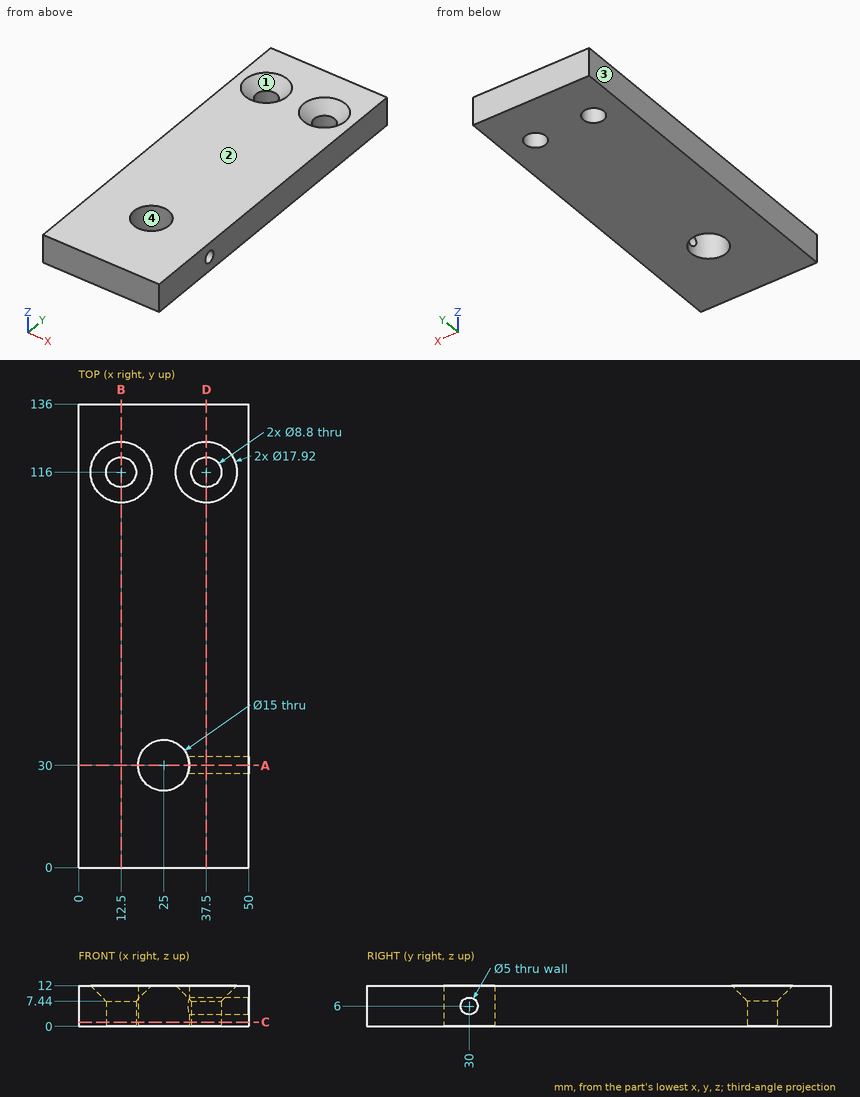
Here's the drawing with two shaded views (mm, measured from the low corner). I have some questions. Round coordinates to 2 decimals unless told otherwise and drop trailing zeros. Order: outer loops, then holes, each group sorted by start corner. A loop starts at its lowest first (then second) coordinate and runs counter-clockwise, first axis right, second up. Notation, with made-up numbers: (-32, 57.25) -> (14, 57.25) arc R25 cw to (14, 90.25) -> close; hole circle Ø1 at (-17, 27). An arc over 180 degrees is marked (long way). Return JSON: item names as keys, results as strings.
Q1. If we section it at A-A on y = 30: List the corners of the cut face in (x, z) for me.
Filled sheet:
{"outline": "(0, 0) -> (17.5, 0) -> (17.5, 12) -> (0, 12) -> close; (32.5, 0) -> (50, 0) -> (50, 3.5) -> (32.5, 3.5) -> close; (32.5, 8.5) -> (50, 8.5) -> (50, 12) -> (32.5, 12) -> close"}
Q2. If we mould it in two halves opening along X, with no side actions, what happens to the marked faces 1, 2, 3 and 4? For each: released by +X, released by -X, zero draft, split by the parting line, or undercut.
Filled sheet:
{"face 1": "undercut", "face 2": "zero draft", "face 3": "released by -X", "face 4": "undercut"}
Q3. If we section it at B-B on x = 12.5: List the corners of the cut face in (y, z) for me.
Filled sheet:
{"outline": "(0, 0) -> (111.6, 0) -> (111.6, 7.44) -> (107.04, 12) -> (0, 12) -> close; (120.4, 0) -> (136, 0) -> (136, 12) -> (124.96, 12) -> (120.4, 7.44) -> close"}
Q4. If we section it at D-D on x = 37.5: List the corners of the cut face in (y, z) for me, plus the area to 3 significant figures.
Filled sheet:
{"outline": "(0, 0) -> (111.6, 0) -> (111.6, 7.44) -> (107.04, 12) -> (0, 12) -> close; (120.4, 0) -> (136, 0) -> (136, 12) -> (124.96, 12) -> (120.4, 7.44) -> close; hole circle Ø5 at (30, 6)", "area": "1,490 mm^2"}
Q5. I need wall thicknesses on line 1 along X through (y, z) = (116, 4); line 2 along Z through (x, y) = (44.5, 30); line 3 along Y through (x, z) = (24.5, 1.75). Which ranges of each line are inside material? Lowest first, please. Write a range as from..to.
Filled sheet:
{"line 1": "x = 0..8.1, 16.9..33.1, 41.9..50", "line 2": "z = 0..3.5, 8.5..12", "line 3": "y = 0..22.52, 37.48..136"}
Q6. If we section it at C-C on z = 1.25: List the corners of the cut face in (x, y) for me.
Filled sheet:
{"outline": "(0, 0) -> (50, 0) -> (50, 136) -> (0, 136) -> close; hole circle Ø8.8 at (12.5, 116); hole circle Ø15 at (25, 30); hole circle Ø8.8 at (37.5, 116)"}
